Geometry: final body of the model. Coordinates: model frame, mm. A direction names the side the tool comes from. Give positions to 0.01 mm unless a question says otherwise; leave off trailing zeros. Loops run counter-clockwise (first coordinate to the right, second up) from the corner with the lowest first, then second, coordinate; pieces in that order, holes last. Notation, with made-up numbers: (69, 13) -> (86, 13) arc R26 cw to (86, 45) -> close; hole circle Ø2 at (-22, 78). An arc over 180 degrees is marked (long way). Answer in a Markdown table with one row per item. Add a question column.
1) Draft query along Y for faces 3 (the cylindrical face through (82.38, 10.71, 5.06)), 4 (the flat face through (43, 0, 7)), 5 (the flat face through (42, 5, 7)). Return one class per face: +Y half, -Y half, draft (parallel to the pull), parting line (faces both ways), or undercut.
2) Section query A-A (z = 7.5). Give the number of separate pieces and of enclosed holes in the cut face, plus the area to 3 significant figures.
3) Section query B-B (y = 19.75). Return the cut outline in (x, z), plus the area to 3 significant figures.
4) Line query: line 1 (Y direction, x = 3.5, z = 7.5); line 2 (X direction, y = 16, z = 10.5); line 3 (Z direction, x = 3.5, y = 11.25). Output: solid intervals per line, ascending. Write a range as from..to.
5) Access query for faces 1 (the cylindrical face through (82.465, 21.766, 5.979)), 2 (the cylindrical face through (6, 7, 7)). Directions: +Z, -Z, +X, -X, +Y, -Y. A direction counts if a zero-diameter tool reaches every point of the face in a straight line with its end or side. Return the directions, or none.
6) First-contact query: P1, Ø8, axis at y = 11.25, z = 7.5, coming from the +X side; P2, Ø4.5, axis at y = 23.75, z = 7.5, coming from the -X side; P3, Ø2, axis at x = 30, z = 6.5, coming from the +Y side. Flat tips, straight axial feed; report the tip coordinate or a pass-through.
7) Section query D-D (x = 18). Return the cut outline in (y, z), plus the area to 3 significant figures.
8) Section query C-C (y = 23.75). Return the cut outline in (x, z).
```python
from build123d import *

# Parameters (mm, degrees)
PAD_DEPTH         = 15
SKETCH001_R       = 2.5
POCKET_DEPTH      = 0.001
POCKET_DEPTH_BACK = -85.001
FILLET_R          = 1


with BuildPart() as part:
    # Sketch → Pad (new body)
    with BuildSketch(Plane.XY):
        with BuildLine():
            Line((85, 30), (85, 0))
            Line((85, 0), (0, 0))
            Line((0, 0), (0, 30))
            Line((0, 30), (5, 30))
            Line((5, 30), (5, 10))
            ThreePointArc((5, 10), (6.464466, 6.464466), (10, 5))
            Line((10, 5), (75, 5))
            ThreePointArc((75, 5), (78.535534, 6.464466), (80, 10))
            Line((80, 10), (80, 30))
            Line((80, 30), (85, 30))
        make_face()
    extrude(amount=PAD_DEPTH)

    # Sketch001 → Pocket (cut, two sides)
    with BuildSketch(Plane.YZ) as pocket_sk:
        with Locations((11.25, 7.5)):
            Circle(SKETCH001_R)
        with Locations((23.75, 7.5)):
            Circle(SKETCH001_R)
    extrude(amount=-POCKET_DEPTH, mode=Mode.SUBTRACT)
    extrude(pocket_sk.sketch, amount=-POCKET_DEPTH_BACK, mode=Mode.SUBTRACT)

    # Fillet
    fillet_edges = [part.edges().sort_by_distance(p)[0] for p in [
        (85, 30, 7.5),
        (80, 30, 7.5),
        (82.5, 30, 0),
        (82.5, 30, 15),
        (85, 0, 7.5),
        (5, 30, 7.5),
        (0, 30, 7.5),
        (0, 0, 7.5),
        (42.5, 0, 15),
        (42.5, 0, 0),
        (85, 15, 15),
        (0, 15, 15),
        (2.5, 30, 15),
        (5, 20, 15),
        (6.464466, 6.464466, 15),
        (42.5, 5, 15),
        (78.535534, 6.464466, 15),
        (80, 20, 15),
        (85, 15, 0),
        (0, 15, 0),
        (2.5, 30, 0),
        (5, 20, 0),
        (6.464466, 6.464466, 0),
        (42.5, 5, 0),
        (78.535534, 6.464466, 0),
        (80, 20, 0),
    ]]
    fillet(fillet_edges, radius=FILLET_R)


solid = part.part
```
Evaluation:
| question | item | result |
|---|---|---|
| 1 | face 3 | undercut |
| 1 | face 4 | -Y half |
| 1 | face 5 | +Y half |
| 2 | separate pieces | 5 |
| 2 | enclosed holes | 0 |
| 2 | area | 584 mm² |
| 3 | outline | (0, 1) arc R1 ccw to (1, 0) -> (4, 0) arc R1 ccw to (5, 1) -> (5, 14) arc R1 ccw to (4, 15) -> (1, 15) arc R1 ccw to (0, 14) -> close; (80, 1) arc R1 ccw to (81, 0) -> (84, 0) arc R1 ccw to (85, 1) -> (85, 14) arc R1 ccw to (84, 15) -> (81, 15) arc R1 ccw to (80, 14) -> close |
| 3 | area | 148 mm² |
| 4 | line 1 | 0..8.75, 13.75..21.25, 26.25..30 |
| 4 | line 2 | 0..5, 80..85 |
| 4 | line 3 | 0..5, 10..15 |
| 5 | face 1 | +X, -X |
| 5 | face 2 | +Z, -Z, +Y |
| 6 | P1 | x = 85 |
| 6 | P2 | through |
| 6 | P3 | y = 5 |
| 7 | outline | (0, 1) arc R1 ccw to (1, 0) -> (4, 0) arc R1 ccw to (5, 1) -> (5, 14) arc R1 ccw to (4, 15) -> (1, 15) arc R1 ccw to (0, 14) -> close |
| 7 | area | 74.1 mm² |
| 8 | outline | (0, 1) arc R1 ccw to (1, 0) -> (4, 0) arc R1 ccw to (5, 1) -> (5, 5) -> (0, 5) -> close; (0, 10) -> (5, 10) -> (5, 14) arc R1 ccw to (4, 15) -> (1, 15) arc R1 ccw to (0, 14) -> close; (80, 1) arc R1 ccw to (81, 0) -> (84, 0) arc R1 ccw to (85, 1) -> (85, 5) -> (80, 5) -> close; (80, 10) -> (85, 10) -> (85, 14) arc R1 ccw to (84, 15) -> (81, 15) arc R1 ccw to (80, 14) -> close |
